Here's how the part is built. I have some questions about the finished solid (model axes, mm). Face numbers are marked on the shaded views. A direction names the side the tool comes from. Give positions to 0.01 mm unless a question says otherwise; leave off trailing zeros. Write each loop counter-clockwise with the first axis right and the second up, starting at its lowest first coordinate (ties: lowest second). Pieces come first, ordered by that corner, then holes. Notation, with made-up numbers: (39.25, -1.5) - (47.25, -1.5) arc R24 ccw to (47.25, 23.5) - close; hole circle Ø7 at (-7, -5). An arc over 180 degrees is marked (long way). Use a Markdown table: item, result.
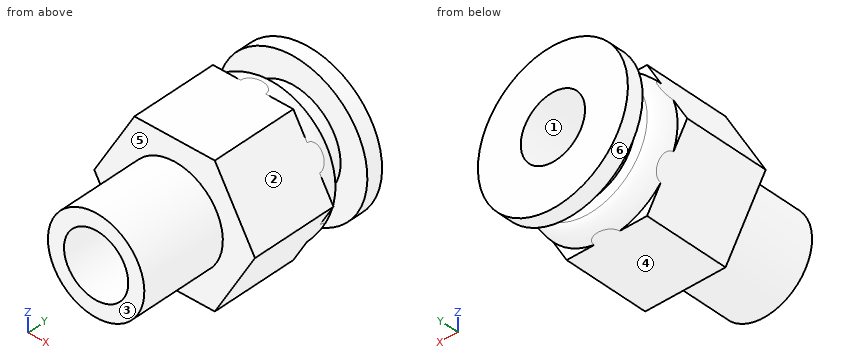
```python
from build123d import *

# Parameters (mm, degrees)
FILLET1_SIZE       = 1
FILLET1_SIZE_2     = 2
CUT_EXTRUDE1_DEPTH = 20.19635382
CIRPATTERN1_COUNT  = 6
SKETCH6_R          = 3
CUT_EXTRUDE2_DEPTH = 21.553284565


with BuildPart() as part:
    # Sketch1 → Revolve1 (revolve)
    with BuildSketch(Plane.XY, mode=Mode.PRIVATE) as revolve1_sk:
        Polygon((0, 10), (6.6, 10), (6.6, 8), (7.5, 8), (7.5, 0), (4.5, 0), (4.5, -8), (0, -8), align=None)
    revolve(revolve1_sk.sketch.rotate(Axis((0, 22.612667954, 0), (0, -1, 0)), 90), axis=Axis((0, 22.612667954, 0), (0, -1, 0)))

    # Fillet1
    # an asymmetric fillet: 2, 1 mm, written as the material it takes off along each edge
    with BuildSketch(Plane(origin=(0, 10, 0), x_dir=(0, 0, 1), z_dir=(1, 0, 0))) as fillet1_piece_1:
        with BuildLine():
            Bezier((6.6 - FILLET1_SIZE, 0), (6.6, 0), (6.6, FILLET1_SIZE_2), weights=[1, 0.707106781, 1])
            Line((6.6, FILLET1_SIZE_2), (6.6, 0))
            Line((6.6, 0), (6.6 - FILLET1_SIZE, 0))
        make_face()
    revolve(axis=Axis((0, 10, 0), (0, -1, 0)), mode=Mode.SUBTRACT)

    # Sketch2 → Cut-Extrude1 (cut, symmetric)
    with BuildSketch(Plane(origin=(0, 8, 0), x_dir=(1, 0, 0), z_dir=(0, 1, 0))):
        with BuildLine():
            Line((3.75, 6.495190528), (7.5, 0))
            ThreePointArc((7.5, 0), (6.495190528, 3.75), (3.75, 6.495190528))
        make_face()
    cut_extrude1 = extrude(amount=CUT_EXTRUDE1_DEPTH, both=True, mode=Mode.SUBTRACT)

    # CirPattern1: Cut-Extrude1 ×6 about axis
    cirpattern1_axis = Axis((0, 0, 0), (0, 1, 0))
    for i in range(1, CIRPATTERN1_COUNT):
        add(cut_extrude1.rotate(cirpattern1_axis, i * 360 / CIRPATTERN1_COUNT), mode=Mode.SUBTRACT)

    # Sketch6 → Cut-Extrude2 (cut, through all)
    with BuildSketch(Plane.XZ.offset(8)):
        with Locations(Location((0, 0, 0), (0, 0, 270))):
            Circle(SKETCH6_R)
    extrude(amount=-CUT_EXTRUDE2_DEPTH, mode=Mode.SUBTRACT)

    # Sketch7 → Revolve2 (revolve)
    with BuildSketch(Plane.XY, mode=Mode.PRIVATE) as revolve2_sk:
        Polygon((3, 10), (3, 13.5), (7, 13.5), (7, 12), (4.5, 12), (4.5, 10), align=None)
    revolve(revolve2_sk.sketch.rotate(Axis((0, 10.01, 0), (0, -1, 0)), 90), axis=Axis((0, 10.01, 0), (0, -1, 0)))


solid = part.part
```
Item 1: Will these pins go through, and if not, where does the flat tip stop? pin 1 Ø1.5 at (x, y) = (6, -4.5) entering from -Z; pin 2 Ø4 at (x, y) = (0, 5.5) entering from +Z; pin 3 Ø1.5 at (y, z) = (10.5, -1.5) entering from +X; pin 4 Ø1 at (x, z) = (-5.5, -4) entering from -Y.
Values:
| item | result |
|---|---|
| pin 1 | passes through |
| pin 2 | stops at z = 6.5 |
| pin 3 | stops at x = 5.92 |
| pin 4 | stops at y = 0 |
Item 2: Thinking about a two-plate mould opening in Z: for the marked faces 1, 2 and 3, which applies, +Z half, -Z half, draft (parallel to the pull), parting line (faces both ways), or undercut?
Values:
| item | result |
|---|---|
| face 1 | undercut |
| face 2 | +Z half |
| face 3 | draft |
Item 3: If we section it at A-A, the plane y = -1.5: Write out the boundary of the cut face in (x, z).
Values:
| item | result |
|---|---|
| outline | circle Ø9 at (0, 0); hole circle Ø6 at (0, 0) |
Item 4: I need wall thicknesses on line 1 along X through (y, z) = (-0.75, 0); line 2 along Y through (x, z) = (5.75, -0.5); line 3 along X through (y, z) = (12.25, 0.5). Which ranges of each line are inside material? Lowest first, please. Write a range as [from, to].
Values:
| item | result |
|---|---|
| line 1 | x = [-4.5, -3], [3, 4.5] |
| line 2 | y = [0, 9.97], [12, 13.5] |
| line 3 | x = [-6.98, -2.96], [2.96, 6.98] |
Item 5: For the marked faces 4, 5 and 6, which set-ups out of +Z, -Z, +X, -X, +Y, -Y let a thin tool reach every point of the face, with its end or its side?
Values:
| item | result |
|---|---|
| face 4 | -Z, +X, -X, -Y |
| face 5 | -Y |
| face 6 | +Y |
